Source: CAD feature listing. Evaluate the final solid. Frame: model axes, mm. Face numbers are marked on the shaded views. A direction names the side the tool comes from. Coordinates: 2 decimals unless noted, no trailing zeros. Write each loop counter-clockwise with the first axis right and the second up, starting at its lowest first coordinate (ties: lowest second). Pieces come first, ordered by that corner, then holes. Notation, with made-up numbers: (76, 15.5) -> (126, 15.5) arc R19 cw to (126, 44.5) -> close; hole circle Ø9 at (-16.75, 9.5). An arc over 180 degrees is marked (long way). One line per item, written item: value. Start each with the question number.
1. First-contact query: P1, Ø0.5, axis at x = 0, z = -0.5, coming from the -Y side; P2, Ø17.5, axis at x = 0, z = 0, coming from the -Y side; P3, Ø1.5, axis at y = -2.5, z = -1.5, coming from the +X side. Flat tips, straight axial feed; report the tip coordinate or a pass-through.
2. Section query B-B, the plane y = -4.75. Output: boundary loops of the cut face in (x, z), and give its area (3 significant figures).
3. Mould query, pull axis X, two halves, no side actions, for the marked faces 1, 2 and 3. Classes: released by +X, released by -X, zero draft, split by the parting line, or undercut.
4. Section query A-A, the plane z = 0. Output: boundary loops of the cut face in (x, y).
5. Line query: line 1 (X direction, y = 4, z = -0.5); line 2 (X direction, y = -3.25, z = 0); line 3 (Z direction, x = 0, y = -0.3). Output: solid intervals per line, ascending.
6. Section query C-C, the plane x = 0. Output: boundary loops of the cut face in (y, z).
7. Access query for the marked faces 4, 5 and 6. Directions: +Z, -Z, +X, -X, +Y, -Y. A direction counts if a zero-diameter tool reaches every point of the face in a straight line with its end or side. Return the directions, or none.
8. Section query D-D, the plane z = -9.5. Output: boundary loops of the cut face in (x, y), and give its area (4 significant figures).
from build123d import *

# Parameters (mm, degrees)
SKETCH_1_R          = 6
SKETCH_1_R_2        = 3.05
EXTRUDE_1_DEPTH     = 9
SKETCH_2_R          = 9
EXTRUDE_2_DEPTH     = 3
SKETCH_3_W          = 0.9
SKETCH_3_H          = 8.759425964
EXTRUDE_3_DEPTH     = 1
EXTRUDE_START       = 10
SKETCH_4_R          = 12.5
SKETCH_4_R_2        = 6
EXTRUDE_4_DEPTH     = 10
EXTRUDE_START_2     = 7
SKETCH_5_R          = 12.5
SKETCH_5_R_2        = 11
EXTRUDE_5_DEPTH     = 7
SKETCH_6_R          = 17.5
SKETCH_6_R_2        = 12.5
EXTRUDE_6_DEPTH     = 20
SKETCH_7_W          = 11.223410854
SKETCH_7_H          = 4
CUT_EXTRUDE_1_DEPTH = 3


with BuildPart() as part:
    # 草图1 → 凸台-拉伸1 (new body)
    with BuildSketch(Plane(origin=(0, 0, 0), x_dir=(1, 0, 0), z_dir=(0, 1, 0))):
        with Locations(Location((0, 0, 0), (0, 0, 270))):
            Circle(SKETCH_1_R)
        with Locations(Location((0, 0, 0), (0, 0, 270))):
            Circle(SKETCH_1_R_2, mode=Mode.SUBTRACT)
    extrude(amount=EXTRUDE_1_DEPTH)

    # 草图2 → 凸台-拉伸2 (add)
    with BuildSketch(Plane(origin=(0, 9, 0), x_dir=(1, 0, 0), z_dir=(0, 1, 0))):
        with Locations(Location((0, 0, 0), (0, 0, 270))):
            Circle(SKETCH_2_R)
    extrude(amount=EXTRUDE_2_DEPTH)

    # 草图3 → 凸台-拉伸3 (add)
    with BuildSketch(Plane.XZ.offset(-9)):
        Rectangle(SKETCH_3_W, SKETCH_3_H)
    extrude(amount=EXTRUDE_3_DEPTH)

    # 草图4 → 凸台-拉伸4 (add)
    with BuildSketch(Plane.XZ.offset(-9).offset(EXTRUDE_START)):
        with Locations(Location((0, 0, 0), (0, 0, 270))):
            Circle(SKETCH_4_R)
        with Locations(Location((0, 0, 0), (0, 0, 90))):
            Circle(SKETCH_4_R_2, mode=Mode.SUBTRACT)
    extrude(amount=-EXTRUDE_4_DEPTH)

    # 草图5 → 凸台-拉伸5 (add)
    with BuildSketch(Plane.XZ.offset(1).offset(EXTRUDE_START_2)):
        with Locations(Location((0, 0, 0), (0, 0, 270))):
            Circle(SKETCH_5_R)
        with Locations(Location((0, 0, 0), (0, 0, 270))):
            Circle(SKETCH_5_R_2, mode=Mode.SUBTRACT)
    extrude(amount=-EXTRUDE_5_DEPTH)

    # 草图6 → 凸台-拉伸6 (add)
    with BuildSketch(Plane.XZ.offset(8)):
        with Locations(Location((0, 0, 0), (0, 0, 270))):
            Circle(SKETCH_6_R)
        with Locations(Location((0, 0, 0), (0, 0, 270))):
            Circle(SKETCH_6_R_2, mode=Mode.SUBTRACT)
    extrude(amount=-EXTRUDE_6_DEPTH)

    # 草图7 → 切除-拉伸1 (cut)
    with BuildSketch(Plane(origin=(0, 12, 0), x_dir=(1, 0, 0), z_dir=(0, 1, 0))):
        with Locations((17.5, 0)):
            Rectangle(SKETCH_7_W, SKETCH_7_H)
    extrude(amount=-CUT_EXTRUDE_1_DEPTH, mode=Mode.SUBTRACT)


solid = part.part
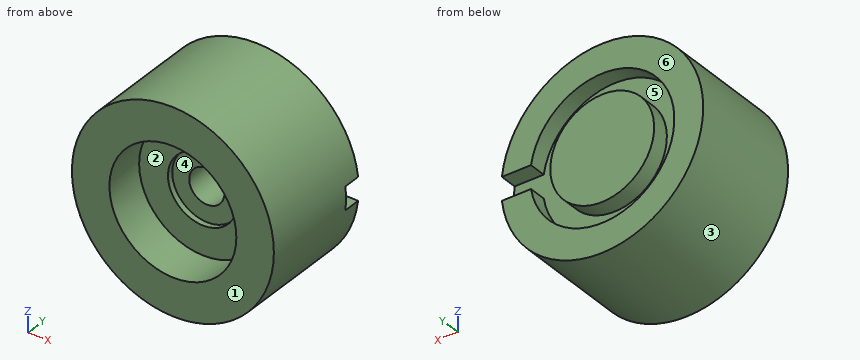
Computed values:
1. P1: stops at y = 8
1. P2: stops at y = -1
1. P3: stops at x = 17.48
2. outline: circle Ø35 at (0, 0); hole circle Ø22 at (0, 0)
2. area: 582 mm²
3. face 1: zero draft
3. face 2: undercut
3. face 3: split by the parting line
4. outline: (-17.5, -8) -> (-11, -8) -> (-11, -1) -> (-6, -1) -> (-6, 0) -> (-3.05, 0) -> (-3.05, 9) -> (-0.45, 9) -> (-0.45, 8) -> (0.45, 8) -> (0.45, 9) -> (3.05, 9) -> (3.05, 0) -> (6, 0) -> (6, -1) -> (11, -1) -> (11, -8) -> (17.5, -8) -> (17.5, 9) -> (9, 9) -> (9, 12) -> (-9, 12) -> (-9, 9) -> (-12.5, 9) -> (-12.5, 12) -> (-17.5, 12) -> close
5. line 1: x = -17.49 to -3.01, 3.01 to 17.49
5. line 2: x = -17.5 to -11, 11 to 17.5
5. line 3: z = -17.5 to -6, 6 to 17.5
6. outline: (-8, -17.5) -> (12, -17.5) -> (12, -12.5) -> (9, -12.5) -> (9, -9) -> (12, -9) -> (12, 9) -> (9, 9) -> (9, 12.5) -> (12, 12.5) -> (12, 17.5) -> (-8, 17.5) -> (-8, 11) -> (-1, 11) -> (-1, 6) -> (0, 6) -> (0, 3.05) -> (8, 3.05) -> (8, -3.05) -> (0, -3.05) -> (0, -6) -> (-1, -6) -> (-1, -11) -> (-8, -11) -> close
7. face 4: -Y
7. face 5: +Y
7. face 6: +Z, -Z, +X, -X, +Y
8. outline: (-14.7, -8) -> (-5.55, -8) -> (-5.55, -1) -> (5.55, -1) -> (5.55, -8) -> (14.7, -8) -> (14.7, 12) -> (8.12, 12) -> (8.12, 9) -> (-8.12, 9) -> (-8.12, 12) -> (-14.7, 12) -> close
8. area: 461.5 mm²
